Input: part model. Units: mm. Frame: model coordinates. Face numbers are marked on the shaded views. A direction names the side the tool comes from. Round coordinates to 2 decimals unless told otherwise and drop trailing zeros. Loops run counter-clockwise (first coordinate to the right, second up) from the corner with the lowest first, then second, coordinate; pieces in that order, holes last. Notation, with made-up numbers: (-2.5, -21) - (50.5, -21) arc R19 cw to (50.5, -14) - close; hole circle Ø11 at (13.25, -30.5). An arc over 180 degrees is marked (long way). One line per question, with ' | ' between items. Start each with the question number.
Item 1: Material intervals for line 1 along X through (y, z) = (6, -3); line 2 along Z through (x, y) = (-60.5, 7.5); line 3 along X through (y, z) = (14.5, 23.5), sorted ascending.
Item 2: Section A-A, the plane y = 25.4. Return loops of the section in (x, z).
Item 3: Section B-B, the plane z = 12.5. Return loops of the section in (x, y).
Item 4: Set-up query: the marked faces 1 and 2. Return all of +Z, -Z, +X, -X, +Y, -Y with unobstructed straight access to the full face (end or side cutting, diameter ignored); none if empty.
Item 5: Section D-D, the plane z = -26. Return loops of the section in (x, y).
Item 6: First-contact query: pin 1 (12 mm diameter, centred on y = 22, z = -9, fed in from +X); pin 2 (10 mm diameter, centred on x = -58, z = 25.5, fed in from +Y); pin 3 (5 mm diameter, centred on y = 19, z = -18.5, fed in from -X); pin 4 (3 mm diameter, centred on x = -24.5, z = 22, fed in from -Y). Flat tips, straight axial feed; report the tip coordinate or a pass-through.
Item 7: Section C-C, the plane y = 48.5. Return loops of the section in (x, z), plus the area to 3 significant figures.
```python
from build123d import *

# Parameters (mm, degrees)
SKETCH1_W           = 104.14
SKETCH1_H           = 88.9
BOSS_EXTRUDE1_DEPTH = 58.42
SKETCH2_W           = 40.64
SKETCH2_H           = 40.64
BOSS_EXTRUDE2_DEPTH = 12.7
SKETCH3_R           = 1.927464999
BOSS_EXTRUDE3_DEPTH = 25.4
SKETCH4_R           = 2.682066204
BOSS_EXTRUDE4_DEPTH = 25.4


with BuildPart() as part:
    # Sketch1 → Boss-Extrude1 (new body)
    with BuildSketch(Plane(origin=(0, 0, 0), x_dir=(1, 0, 0), z_dir=(0, 1, 0))):
        Rectangle(SKETCH1_W, SKETCH1_H)
    extrude(amount=BOSS_EXTRUDE1_DEPTH)

    # Sketch2 → Boss-Extrude2 (add)
    with BuildSketch(Plane.ZY.offset(52.07)):
        with Locations((20.544561746, 20.32)):
            Rectangle(SKETCH2_W, SKETCH2_H)
    extrude(amount=BOSS_EXTRUDE2_DEPTH)

    # Sketch3 → Boss-Extrude3 (add)
    with BuildSketch(Plane(origin=(52.07, 0, 0), x_dir=(0, 0, -1), z_dir=(1, 0, 0))):
        with Locations(Location((-16.51, 25.4, 0), (0, 0, 180))):
            Circle(SKETCH3_R)
    extrude(amount=BOSS_EXTRUDE3_DEPTH)

    # Sketch4 → Boss-Extrude4 (add)
    with BuildSketch(Plane.ZY.offset(52.07)):
        with Locations(Location((-39.37, 25.4, 0), (0, 0, 180))):
            Circle(SKETCH4_R)
    extrude(amount=BOSS_EXTRUDE4_DEPTH)


solid = part.part
```
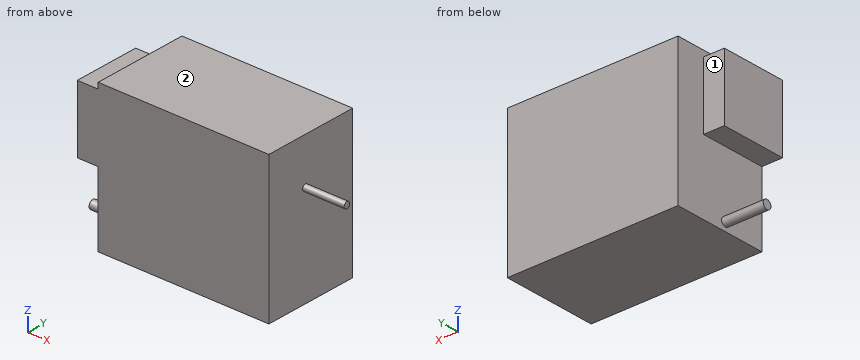
Return value:
1) line 1: -52.07 to 52.07 | line 2: 0.22 to 40.86 | line 3: -64.77 to 52.07
2) outline: (-77.47, -42.05) - (-52.07, -42.05) - (-52.07, -44.45) - (52.07, -44.45) - (52.07, 14.58) - (77.47, 14.58) - (77.47, 18.44) - (52.07, 18.44) - (52.07, 44.45) - (-52.07, 44.45) - (-52.07, 40.86) - (-64.77, 40.86) - (-64.77, 0.22) - (-52.07, 0.22) - (-52.07, -36.69) - (-77.47, -36.69) - close
3) outline: (-64.77, 0) - (52.07, 0) - (52.07, 58.42) - (-52.07, 58.42) - (-52.07, 40.64) - (-64.77, 40.64) - close
4) face 1: +Z, -Z, -X, +Y | face 2: +Z, +X, -X, +Y, -Y
5) outline: (-52.07, 0) - (52.07, 0) - (52.07, 58.42) - (-52.07, 58.42) - close
6) pin 1: x = 52.07 | pin 2: y = 40.64 | pin 3: x = -52.07 | pin 4: y = 0
7) outline: (-52.07, -44.45) - (52.07, -44.45) - (52.07, 44.45) - (-52.07, 44.45) - close | area: 9,260 mm2
